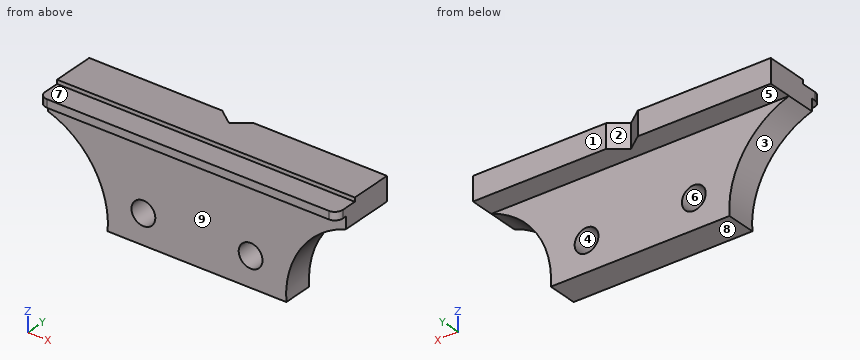
from build123d import *

# Parameters (mm, degrees)
F1_DEPTH      = 75
F4_DEPTH      = 25
F4_DEPTH_BACK = 25
F5_R          = 3
F6_DEPTH      = 25
F6_DEPTH_BACK = 25
F7_R          = 2
F9_DEPTH      = 50


with BuildPart() as f1:
    # F0 (on Right) → F1 (new body)
    with BuildSketch(Plane.YZ):
        Polygon((-7.5, 0), (0, 0), (0, 22.5), (6, 22.5), (6, 28.5), (-4.5733697172, 28.5), (-4.5733697172, 27.5), (-10.5, 27.5), (-10.5, 25.5), (-7.5, 25.5), align=None)
    extrude(amount=F1_DEPTH)

    # F2 (on Front) → F4 (cut, two sides)
    with BuildSketch(Plane.XZ) as f4_sk:
        with BuildLine():
            Line((18.9505368471, -15.0200538337), (15, 0))
            ThreePointArc((15, 0), (11.3650779756, 13.8267186504), (0, 22.5))
            Line((0, 22.5), (-15.862300992, 22.5))
            Line((-15.862300992, 22.5), (-15.862300992, -15.0200538337))
            Line((-15.862300992, -15.0200538337), (18.9505368471, -15.0200538337))
        make_face()
        with BuildLine():
            Line((90.862300992, 22.5), (75, 22.5))
            ThreePointArc((75, 22.5), (63.6349220244, 13.8267186504), (60, 0))
            Line((60, 0), (56.0494631529, -15.0200538337))
            Line((56.0494631529, -15.0200538337), (90.862300992, -15.0200538337))
            Line((90.862300992, -15.0200538337), (90.862300992, 22.5))
        make_face()
    extrude(amount=-F4_DEPTH, mode=Mode.SUBTRACT)
    extrude(f4_sk.sketch, amount=F4_DEPTH_BACK, mode=Mode.SUBTRACT)

    # F5 (on Front) → F6 (cut, two sides)
    with BuildSketch(Plane.XZ) as f6_sk:
        with Locations((24, 7.5)):
            Circle(F5_R)
        with Locations((51, 7.5)):
            Circle(F5_R)
    extrude(amount=F6_DEPTH, mode=Mode.SUBTRACT)
    extrude(f6_sk.sketch, amount=-F6_DEPTH_BACK, mode=Mode.SUBTRACT)

    # F7
    f7_edges = [f1.edges().sort_by_distance(p)[0] for p in [
        (75, -10.5, 26.5),
        (0, -10.5, 26.5),
    ]]
    fillet(f7_edges, radius=F7_R)

    # F8 (on Top) → F9 (cut)
    with BuildSketch(Plane.XY):
        Polygon((32.4930176139, 11.9444662705), (33.5, 6), (37.5, 3), (41.5, 6), (50.5435075659, 15.0021882955), align=None)
    extrude(amount=F9_DEPTH, mode=Mode.SUBTRACT)


solid = f1.part
Build history of the part. All positions in model axes, mm. Face numbers are marked on the shaded views. A direction names the side the tool comes from. Coordinates: 2 decimals unless noted, no trailing zeros. Write each loop counter-clockwise with the first axis right and the second up, starting at its lowest first coordinate (ties: lowest second). Pieces come first, ordered by that corner, then holes.
(1) Cut at D-D on z = 8.75. List the corners of the cut face in (x, y), and give its area (3 significant figures).
(2) Cut at A-A on x = 51. List the corners of the cut face in (y, z).
(3) Drill centre lines: line 1 (Z direction, x = 24, y = -5); line 2 (Z direction, x = 51, y = -3.25); line 3 (X direction, y = -3.25, z = 7.5). Where is each one in solid material? Low to high.
(4) Cut at B-B on y = 4.5. List the corners of the cut face in (x, z).
(5) Mould opens along X. For the marked faces 1, 2, 3 and 4 say: pulls with the +X half, pulls with the -X half, needs draft (parallel to the pull), parting line crosses it, or undercut.
(6) Cut at C-C on z = 23.75. List the corners of the cut face in (x, y), and give its area (3 significant figures).
(7) 3-axis set-ups, long thin cutter, end or side, ignore diameter. For the marked faces 5, 6, 7, 8 and 9: which of +Z, -Z, +X, -X, +Y, -Y reach the whole face in a straight line?
(8) Pin check, flat tips, straight feed: pin 1 Ø0.9 at (x, y) = (30, -9.5) entering from -Z; pin 2 Ø8 at (x, z) = (24, 7.5) entering from +Y; pin 3 Ø7.5 at (x, z) = (49.5, 9.5) entering from -Y. Stop position of each tip, or through.
Working result:
1. outline: (13.87, -7.5) - (21.27, -7.5) - (21.27, 0) - (13.87, 0) - close; (26.73, -7.5) - (48.27, -7.5) - (48.27, 0) - (26.73, 0) - close; (53.73, -7.5) - (61.13, -7.5) - (61.13, 0) - (53.73, 0) - close
1. area: 273 mm2
2. outline: (-10.5, 25.5) - (-7.5, 25.5) - (-7.5, 10.5) - (0, 10.5) - (0, 22.5) - (6, 22.5) - (6, 28.5) - (-4.57, 28.5) - (-4.57, 27.5) - (-10.5, 27.5) - close; (-7.5, 0) - (0, 0) - (0, 4.5) - (-7.5, 4.5) - close
3. line 1: z = 0 to 4.5, 10.5 to 27.5
3. line 2: z = 0 to 4.5, 10.5 to 28.5
3. line 3: x = 14.26 to 21, 27 to 48, 54 to 60.74
4. outline: (0, 22.5) - (35.5, 22.5) - (35.5, 28.5) - (0, 28.5) - close; (39.5, 22.5) - (75, 22.5) - (75, 28.5) - (39.5, 28.5) - close
5. face 1: needs draft
5. face 2: undercut
5. face 3: pulls with the -X half
5. face 4: undercut
6. outline: (0, -7.5) - (75, -7.5) - (75, 6) - (41.5, 6) - (37.5, 3) - (33.5, 6) - (0, 6) - close
6. area: 1,000 mm2
7. face 5: -Z, +X, -X, +Y
7. face 6: +Y, -Y
7. face 7: +Z, +X, -X, -Y
7. face 8: -Z, +X, -X, +Y, -Y
7. face 9: -Z, +X, -X, -Y
8. pin 1: stops at z = 25.5
8. pin 2: stops at y = 0
8. pin 3: stops at y = -7.5
